For this review, take the finished solid that the model builds, in its own axes (mm). Round coordinates to 2 decimals unless told otherwise and drop trailing zeros. Loops run counter-clockwise (first coordinate to the right, second up) from the corner with the lowest first, then second, coordinate; pieces in that order, holes last.
1. Consider section A-A on z = 17.5. State the section outline as (x, y) points, then the cut area to 3 significant figures.
2. Consider section B-B on x = 13. State the section outline as (y, z) points.
3. Clearance check with flat-ended pins moving along their axes: pin 1 Ø10 at (y, z) = (18, 15) entering from -X; pin 2 Ø8 at (y, z) = (22, 16) entering from -X; pin 3 Ø10 at (y, z) = (35, 15.5) entering from -X. State where each tip first meets the part, or that it passes through.
4. Consider section C-C on y = 9. State how many separate pieces and enclosed holes the cut face has, then the cut area to 3 significant figures.
5. To check wall thickness, follow line 1 along Z through (x, y) = (30, 14); line 2 along Z through (x, y) = (46.5, 28); line 3 along Y through (x, z) = (13, 28.5). State the ranges of each line that lie inside material, in increasing order.
from build123d import *

# Parameters (mm, degrees)
EXTRUDE_1_DEPTH     = 60
SKETCH_2_R          = 0.85
CUT_EXTRUDE_1_DEPTH = 30


with BuildPart() as part:
    # 草图1 → 凸台-拉伸1 (new body)
    with BuildSketch(Plane.XY):
        Polygon((0, 0), (70, 0), (70, 43.414518843), (0, 3), align=None)
    extrude(amount=EXTRUDE_1_DEPTH)

    # 草图2 → 切除-拉伸1 (cut, symmetric)
    with BuildSketch(Plane(origin=(-1.299038106, 2.25, 0), x_dir=(0.8660254037844386, 0.5, 0), z_dir=(-0.5000000000000001, 0.8660254037844387, 0))):
        with Locations(Location((32.793518843, -19.503, 0), (0, 0, 180))):
            Circle(SKETCH_2_R)
        with Locations(Location((53.801518843, -23.123, 0), (0, 0, 180))):
            Circle(SKETCH_2_R)
        with Locations(Location((49.374518843, -40.502, 0), (0, 0, 180))):
            Circle(SKETCH_2_R)
        with Locations(Location((31.173518843, -37.391, 0), (0, 0, 180))):
            Circle(SKETCH_2_R)
    extrude(amount=CUT_EXTRUDE_1_DEPTH, both=True, mode=Mode.SUBTRACT)


solid = part.part
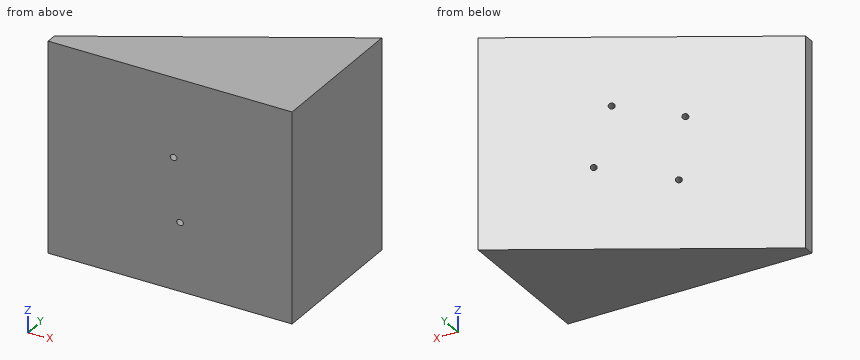
Resolved:
1. outline: (0, 0) - (70, 0) - (70, 43.41) - (0, 3) - close
1. area: 1,620 mm2
2. outline: (0, 0) - (10.51, 0) - (10.51, 60) - (0, 60) - close
3. pin 1: stops at x = 17.32
3. pin 2: stops at x = 25.98
3. pin 3: stops at x = 46.77
4. separate pieces: 1
4. enclosed holes: 4
4. area: 3,570 mm2
5. line 1: z = 0 to 18.67, 20.33 to 60
5. line 2: z = 0 to 22.41, 23.83 to 60
5. line 3: y = 0 to 10.51
